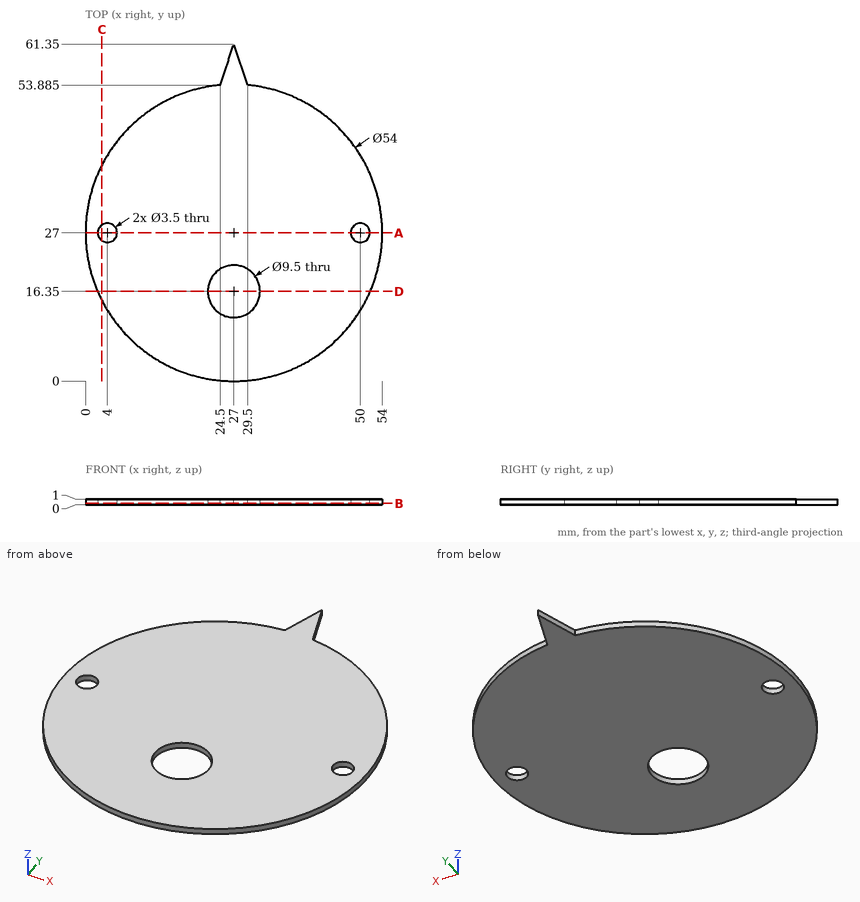
Input: dimensioned drawing with shaded views. Units: mm. Origin: part minimum x, y, z. Coordinates: 2 decimals unless noted, no trailing zeros. Order: outer loops, then holes, each group sorted by start corner. A loop starts at its lowest first (then second) coordinate and runs counter-clockwise, first axis right, second up. Notation, with made-up numbers: M 75,43 L 107,43 A26 ccw 107,72 Z; hole C -3.5,37 d3. An arc over 180 degrees is marked long. Write each question's results on one line, items separated by ' | '. Start each with the question number.
Item 1: Line query: probe 1 along Y at (x, z) = (4, 0.6); probe 2 along X at (y, z) = (40, 0.2); probe 3 along Y at (x, z) = (10, 0.1). Output: solid intervals per line, ascending.
Item 2: Cut plane A-A (y = 27). Return loops of the section in (x, z), and give its area (3 significant figures).
Item 3: Cut plane D-D (y = 16.35). Return loops of the section in (x, z).
Item 4: Cut plane B-B (z = 0.25). Count the separate pieces of the cut face and the enclosed holes in it, and give its area (3 significant figures).
Item 5: Cut plane C-C (x = 3). Return loops of the section in (y, z), and give its area (3 significant figures).
Checked values:
1) probe 1: y = 12.86 to 25.25, 28.75 to 41.14 | probe 2: x = 3.34 to 50.66 | probe 3: y = 6.02 to 47.98
2) outline: M 0,0 L 2.25,0 L 2.25,1 L 0,1 Z; M 5.75,0 L 48.25,0 L 48.25,1 L 5.75,1 Z; M 51.75,0 L 54,0 L 54,1 L 51.75,1 Z | area: 47.0 mm2
3) outline: M 2.19,0 L 22.25,0 L 22.25,1 L 2.19,1 Z; M 31.75,0 L 51.81,0 L 51.81,1 L 31.75,1 Z
4) separate pieces: 1 | enclosed holes: 3 | area: 2,220 mm2
5) outline: M 14.63,0 L 25.56,0 L 25.56,1 L 14.63,1 Z; M 28.44,0 L 39.37,0 L 39.37,1 L 28.44,1 Z | area: 21.9 mm2
